Geometry check sheet. Reference: the model listing, model coordinates, mm. Give positions to 0.01 mm unless a question says otherwise; leave off trailing zeros. Write each loop counter-clockwise with the first axis right and the second up, starting at its lowest first coordinate (ties: lowest second). Pieces come first, ordered by that corner, then holes.
(1) Mould release check, pull along X, two halves, no side actions. Record for faces 1 (the flat face through (57.5, 3, 0)), 2 (the flat face through (-1, 3, -30)), 3 (the cylindrical face through (48.103, 3.057, 16.21)): +X half, -X half, draft (parallel to the pull), parting line (faces both ways), or undercut.
(2) Cross-section at D-D (y = 1.25). Record the boundary of the cut face in (x, z).
(3) Cross-section at B-B (z = 4). Record the boundary of the cut face in (x, y), and give its area (3 significant figures).
(4) Thickness scan on line 1 along X through (y, z) = (3.5, -15); line 2 along Z through (x, y) = (50, 1.75); line 3 along Z through (x, y) = (-1.5, 4). Record the ranges inside material, lowest first.
(5) Cross-section at A-A (x = 0). Record the boundary of the cut face in (y, z).
(6) Cross-section at C-C (z = -15). Record the boundary of the cut face in (x, y), and give its area (3 significant figures).
Autodesk Inventor part; units mm, degrees
ref_plane "YZ Plane" through (0, 0, 0) normal (1, 0, 0) x (0, 1, 0)
ref_plane "XZ Plane" through (0, 0, 0) normal (0, 1, 0) x (-1, 0, 0)
ref_plane "XY Plane" through (0, 0, 0) normal (0, 0, 1) x (1, 0, 0)
sketch "Sketch1" plane through (0, 0, 0) normal (0, 1, 0) x (-1, 0, 0)
  line L0 (57.5, -30) -> (-57.5, -30)
  line L1 (-57.5, -30) -> (-57.5, 30)
  line L2 (-57.5, 30) -> (57.5, 30)
  line L3 (57.5, 30) -> (57.5, -30)
  line L4 (57.5, -30) -> (-57.5, 30) construction
  line L5 (-57.5, -30) -> (57.5, 30) construction
  point P0 (0, 0)
  dimension "d0" = 115
  dimension "d1" = 60
extrude "Extrusion1" add sketch "Sketch1" along normal blind 6.2
sketch "Sketch2" plane through (0, 6.2, 0) normal (0, 1, 0) x (1, 0, 0)
  line L0 (57.5, 30) -> (-57.5, 30)
  line L1 (-57.5, 30) -> (-57.5, -30)
  line L2 (-57.5, -30) -> (57.5, -30)
  line L3 (57.5, -30) -> (57.5, 30)
  point P0 (0, 0)
  point P1 (-50, -15)
  point P2 (-50, 15)
  point P3 (50, -15)
  point P4 (50, 15)
  dimension "d4" = 15
  dimension "d5" = 7.5
  dimension "d6" = 15
  dimension "d7" = 7.5
hole "Hole1" at (-50, 6.2, 15) at (-50, 6.2, -15) at (50, 6.2, 15) at (50, 6.2, -15) direction (0, -1, 0) diameter 4.5 end through all
sketch "Sketch3" plane through (0, 6.2, 0) normal (0, 1, 0) x (1, 0, 0)
  point P0 (0, 0)
  point P1 (0, -5)
  point P2 (0, 5)
  dimension "d15" = 5
  dimension "d16" = 5
hole "Hole2" at (0, 6.2, 5) at (0, 6.2, -5) direction (0, -1, 0) diameter 5.2 end through all
properties part number "AjusteBalancin"
Reply:
1. face 1: +X half
1. face 2: draft
1. face 3: undercut
2. outline: (-57.5, -30) - (57.5, -30) - (57.5, 30) - (-57.5, 30) - close; hole circle Ø4.5 at (-50, -15); hole circle Ø4.5 at (-50, 15); hole circle Ø5.2 at (0, -5); hole circle Ø5.2 at (0, 5); hole circle Ø4.5 at (50, -15); hole circle Ø4.5 at (50, 15)
3. outline: (-57.5, 0) - (-2.4, 0) - (-2.4, 6.2) - (-57.5, 6.2) - close; (2.4, 0) - (57.5, 0) - (57.5, 6.2) - (2.4, 6.2) - close
3. area: 683 mm2
4. line 1: x = -57.5 to -52.25, -47.75 to 47.75, 52.25 to 57.5
4. line 2: z = -30 to -17.25, -12.75 to 12.75, 17.25 to 30
4. line 3: z = -30 to -7.12, -2.88 to 2.88, 7.12 to 30
5. outline: (0, -30) - (6.2, -30) - (6.2, -7.6) - (0, -7.6) - close; (0, -2.4) - (6.2, -2.4) - (6.2, 2.4) - (0, 2.4) - close; (0, 7.6) - (6.2, 7.6) - (6.2, 30) - (0, 30) - close
6. outline: (-57.5, 0) - (-52.25, 0) - (-52.25, 6.2) - (-57.5, 6.2) - close; (-47.75, 0) - (47.75, 0) - (47.75, 6.2) - (-47.75, 6.2) - close; (52.25, 0) - (57.5, 0) - (57.5, 6.2) - (52.25, 6.2) - close
6. area: 657 mm2
